Autodesk Inventor part; units mm, degrees
ref_plane "YZ Plane" through (0, 0, 0) normal (1, 0, 0) x (0, 1, 0)
ref_plane "XZ Plane" through (0, 0, 0) normal (0, 1, 0) x (-1, 0, 0)
ref_plane "XY Plane" through (0, 0, 0) normal (0, 0, 1) x (1, 0, 0)
sketch "Sketch2" plane through (0, 0, 0) normal (0, 1, 0) x (-1, 0, 0)
  line L0 (85, 85) -> (-85, 85)
  line L1 (-85, 85) -> (-85, -85)
  line L2 (-85, -85) -> (85, -85)
  line L3 (85, -85) -> (85, 85)
  line L4 (85, 0) -> (-85, 0) construction
  line L5 (0, 85) -> (0, -85) construction
  line L6 (83, 83) -> (47.7, 83)
  line L7 (47.7, 83) -> (47.7, 62.7)
  line L8 (47.7, 62.7) -> (83, 62.7)
  line L9 (83, 62.7) -> (83, 83)
  line L10 (83, 41.7) -> (47.7, 41.7)
  line L11 (47.7, 41.7) -> (47.7, 21.4)
  line L12 (47.7, 21.4) -> (83, 21.4)
  line L13 (83, 21.4) -> (83, 41.7)
  circle A0 centre (74, 74) radius 1.5
  circle A1 centre (57, 74) radius 1.5
  circle A2 centre (74, 30.4) radius 1.5
  circle A3 centre (57, 30.4) radius 1.5
  line L14 (83, -83) -> (47.7, -83)
  line L15 (47.7, -83) -> (47.7, -62.7)
  line L16 (47.7, -62.7) -> (83, -62.7)
  line L17 (83, -62.7) -> (83, -83)
  line L18 (83, -41.7) -> (47.7, -41.7)
  line L19 (47.7, -41.7) -> (47.7, -21.4)
  line L20 (47.7, -21.4) -> (83, -21.4)
  line L21 (83, -21.4) -> (83, -41.7)
  circle A4 centre (74, -74) radius 1.5
  circle A5 centre (57, -74) radius 1.5
  circle A6 centre (74, -30.4) radius 1.5
  circle A7 centre (57, -30.4) radius 1.5
  line L22 (-83, 83) -> (-47.7, 83)
  line L23 (-47.7, 83) -> (-47.7, 62.7)
  line L24 (-47.7, 62.7) -> (-83, 62.7)
  line L25 (-83, 62.7) -> (-83, 83)
  line L26 (-83, 41.7) -> (-47.7, 41.7)
  line L27 (-47.7, 41.7) -> (-47.7, 21.4)
  line L28 (-47.7, 21.4) -> (-83, 21.4)
  line L29 (-83, 21.4) -> (-83, 41.7)
  circle A8 centre (-74, 74) radius 1.5
  circle A9 centre (-57, 74) radius 1.5
  circle A10 centre (-74, 30.4) radius 1.5
  circle A11 centre (-57, 30.4) radius 1.5
  line L30 (-47.7, -62.7) -> (-83, -62.7)
  circle A12 centre (-57, -74) radius 1.5
  circle A13 centre (-74, -74) radius 1.5
  line L31 (-47.7, -83) -> (-47.7, -62.7)
  line L32 (-83, -83) -> (-47.7, -83)
  line L33 (-83, -62.7) -> (-83, -83)
  line L34 (-83, -41.7) -> (-47.7, -41.7)
  circle A14 centre (-57, -30.4) radius 1.5
  circle A15 centre (-74, -30.4) radius 1.5
  line L35 (-83, -21.4) -> (-83, -41.7)
  line L36 (-47.7, -41.7) -> (-47.7, -21.4)
  line L37 (-47.7, -21.4) -> (-83, -21.4)
  circle A16 centre (-82, 17.4) radius 1.5
  circle A17 centre (-82, -17.4) radius 1.5
  circle A18 centre (82, 17.4) radius 1.5
  circle A19 centre (82, -17.4) radius 1.5
  circle A20 centre (-47.7, 17.4625) radius 1.5
  circle A21 centre (-47.7, -17.4) radius 1.5
  circle A22 centre (47.7, 17.4625) radius 1.5
  circle A23 centre (47.7, -17.4) radius 1.5
  point P0 (0, 0)
  point P1 (83, 72.85)
  point P2 (65.35, 83)
  point P3 (83, -72.85)
  point P4 (65.35, -83)
  point P5 (-83, 72.85)
  point P6 (-65.35, 83)
  point P7 (-83, -72.85)
  point P8 (-65.35, -83)
  dimension "d17" = 170
  dimension "d18" = 170
  dimension "d19" = 35.3
  dimension "d20" = 20.3
  dimension "d21" = 2
  dimension "d22" = 2
  dimension "d23" = 20.3
  dimension "d24" = 21
  dimension "d25" = 3
  dimension "d26" = 9
  dimension "d27" = 9
  dimension "d28" = 3
  dimension "d29" = 17
  dimension "d30" = 3
  dimension "d31" = 9
  dimension "d32" = 9
  dimension "d33" = 3
  dimension "d38" = 3
  dimension "d39" = 3
  dimension "d40" = 4
  dimension "d41" = 34.8
  dimension "d44" = 3
  dimension "d45" = 3
  dimension "d46" = 34.3
extrude "Extrusion3" add sketch "Sketch2" along normal blind 5 contours L3 L2 L1 L0 | A16 | A17 | A18 | A19 | A20 | A21 | A22 | A23
extrude "Extrusion4" add sketch "Sketch2" along normal blind 3 contours L9 L8 L7 L6 | L13 L12 L11 L10 | L14 L15 L16 L17 | L18 L19 L20 L21 | L22 L23 L24 L25 | L26 L27 L28 L29 | L31 L32 L33 L30 | L35 L37 L36 L34
extrude "Extrusion5" cut sketch "Sketch2" along normal blind 5 contours A16 | A17 | A18 | A19
extrude "Extrusion6" cut sketch "Sketch2" along normal blind 5 contours A20 | A21 | A22 | A23
properties part number "Casis"
Geometry check sheet. Reference: the model listing, model coordinates, mm. A direction names the side the tool comes from. Coordinates: 2 decimals unless noted, no trailing zeros. Loops run counter-clockwise (first coordinate to the right, second up) from the corner with the lowest first, then second, coordinate; pieces in that order, holes last. Notation, with made-up numbers: (-14.75, -32) -> (22.25, -32) arc R7 cw to (22.25, -23) -> close; hole circle Ø5 at (-12.5, 21). An arc over 180 degrees is marked (long way). Put each result on its own line as item: value.
1) Gauge pin test, flat end, axial feed: pin 1 Ø4 at (x, z) = (-57, -74) entering from -Y. Record the tip position at first contact, or that the pin passes through.
Result set:
pin 1: stops at y = 0
2) Tool access check on faces 5 (the flat face through (1, 0, 1)), 6 (the flat face through (-65, 3, 32)). Record the directions out of +Z, -Z, +X, -X, +Y, -Y that give a thin tool (end or side, any length) a straight path to the whole face; none if there is none.
Result set:
face 5: +Z, -Z, +X, -X, -Y
face 6: +Y
3) Cross-section at B-B on y = 4.2. Count the separate pieces of the cut face and the enclosed holes in it, plus the area to 3 significant figures.
Result set:
separate pieces: 1
enclosed holes: 16
area: 23,100 mm^2
4) Release check for a two-part mould opening along X. For faces 1 (the flat face through (66, 3, -31)), 2 (the flat face through (85, 2, 1)), 3 (the flat face through (-85, 2, -1)), 4 (the flat face through (1, 2, -85)) record: released by +X, released by -X, zero draft, split by the parting line, or undercut.
Result set:
face 1: undercut
face 2: released by +X
face 3: released by -X
face 4: zero draft
5) Cross-section at A-A on z = -34. Record the boundary of the cut face in (x, y), plus the area to 3 significant figures.
Result set:
outline: (-85, 0) -> (85, 0) -> (85, 5) -> (83, 5) -> (83, 3) -> (47.7, 3) -> (47.7, 5) -> (-47.7, 5) -> (-47.7, 3) -> (-83, 3) -> (-83, 5) -> (-85, 5) -> close
area: 709 mm^2
6) Thickness scan on line 1 (Z direction, x = 74, y = 2.3); line 2 (X direction, y = 3.2, z = 41.5); line 3 (Z direction, x = -62, y = 4.7). Record the ranges inside material, lowest first.
Result set:
line 1: z = -85 to -75.5, -72.5 to -31.9, -28.9 to 28.9, 31.9 to 72.5, 75.5 to 85
line 2: x = -85 to -83, -47.7 to 47.7, 83 to 85
line 3: z = -85 to -83, -62.7 to -41.7, -21.4 to 21.4, 41.7 to 62.7, 83 to 85
